The drawing under review shows one solid part. Ordinate dimensions are in mm from its lowest x, y, z. A direction names the side the tool comes from. Round coordinates to 2 decimals unless told otherwise and drop trailing zeros. Order: outer loops, then holes, each group sorted by start corner. A loop starts at its lowest first (then second) coordinate and runs counter-clockwise, first axis right, second up. Notation, with made-up numbers: (-32, -5.5) - (3, -5.5) arc R34 cw to (3, 33.5) - close; hole circle Ø4 at (-24.5, 75.25). An arc over 180 degrees is marked (long way). One line per question, with ' | ' between items.
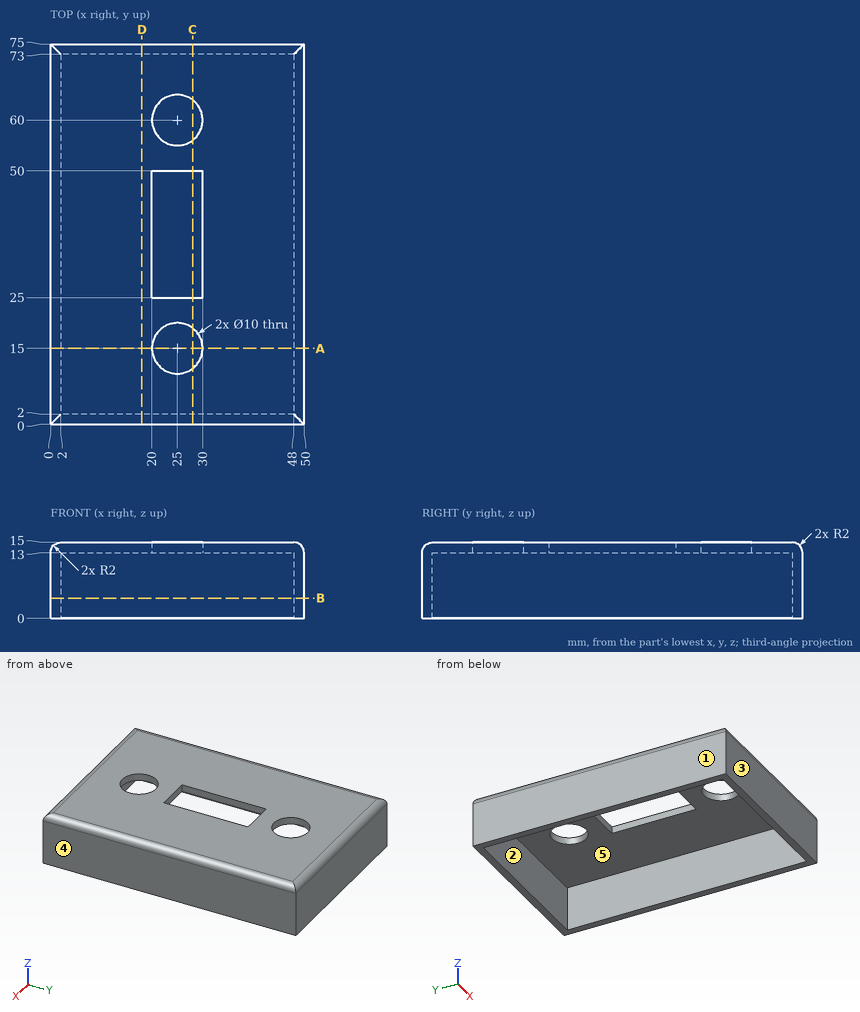
(1) We need section B-B on z = 4. State the section outline as (x, y) points, plus the area to 3 significant figures.
Output values:
outline: (0, 0) - (50, 0) - (50, 75) - (0, 75) - close; hole (2, 2) - (48, 2) - (48, 73) - (2, 73) - close | area: 484 mm^2
(2) We need section A-A on y = 15. State the section outline as (x, z) points, plus the area to 3 significant figures.
Output values:
outline: (0, 0) - (2, 0) - (2, 13) - (20, 13) - (20, 15) - (2, 15) arc R2 ccw to (0, 13) - close; (30, 13) - (48, 13) - (48, 0) - (50, 0) - (50, 13) arc R2 ccw to (48, 15) - (30, 15) - close | area: 130 mm^2
(3) Mouldability with a two-part tool opening along Y and no side actions: class the marked faces 1, 2 and 3 as released by +Y, released by -Y, zero draft, split by the parting line, or undercut.
Output values:
face 1: zero draft | face 2: undercut | face 3: released by -Y
(4) We need section D-D on x = 18. State the section outline as (y, z) points.
Output values:
outline: (0, 0) - (2, 0) - (2, 13) - (73, 13) - (73, 0) - (75, 0) - (75, 13) arc R2 ccw to (73, 15) - (2, 15) arc R2 ccw to (0, 13) - close
(5) For probe 1 along X at (y, z) = (18.5, 4.75); probe 2 along Y at (x, z) = (38, 3.25); probe 3 along Y at (x, z) = (25, 14.15), list the stretches that pass through material, from the lowest coordinate up. Write a range as [from, to].
Output values:
probe 1: [0, 2], [48, 50] | probe 2: [0, 2], [73, 75] | probe 3: [0.36, 10], [20, 25], [50, 55], [65, 74.64]
(6) Insertion check: pin 1 (2 mm diameter, centred on y = 31.5, z = 14.5, fed in from +X); pin 2 (8 mm diameter, centred on x = 25, y = 15, fed in from -Z); pin 3 (5 mm diameter, centred on x = 27, y = 62.5, fed in from +Z); pin 4 (1.6 mm diameter, centred on x = 27.5, z = 14.5, fed in from -Y). Each pin has a flat end and moves straight along its axis. Give the tip position at first contact, or say it passes through.
Output values:
pin 1: x = 49.94 | pin 2: through | pin 3: z = 15 | pin 4: y = 0.13
(7) For the marked faces 4 and 5, list the 3-axis set-ups (+Z, -Z, +X, -X, +Y, -Y) from which the entire face can be reached by the end or side of a thin tool; tool diameter is ignored.
Output values:
face 4: +Z, -Z, +X, +Y, -Y | face 5: -Z
(8) We need section C-C on x = 28. State the section outline as (y, z) points, plus the area to 3 significant figures.
Output values:
outline: (0, 0) - (2, 0) - (2, 13) - (11, 13) - (11, 15) - (2, 15) arc R2 ccw to (0, 13) - close; (19, 13) - (25, 13) - (25, 15) - (19, 15) - close; (50, 13) - (56, 13) - (56, 15) - (50, 15) - close; (64, 13) - (73, 13) - (73, 0) - (75, 0) - (75, 13) arc R2 ccw to (73, 15) - (64, 15) - close | area: 118 mm^2
